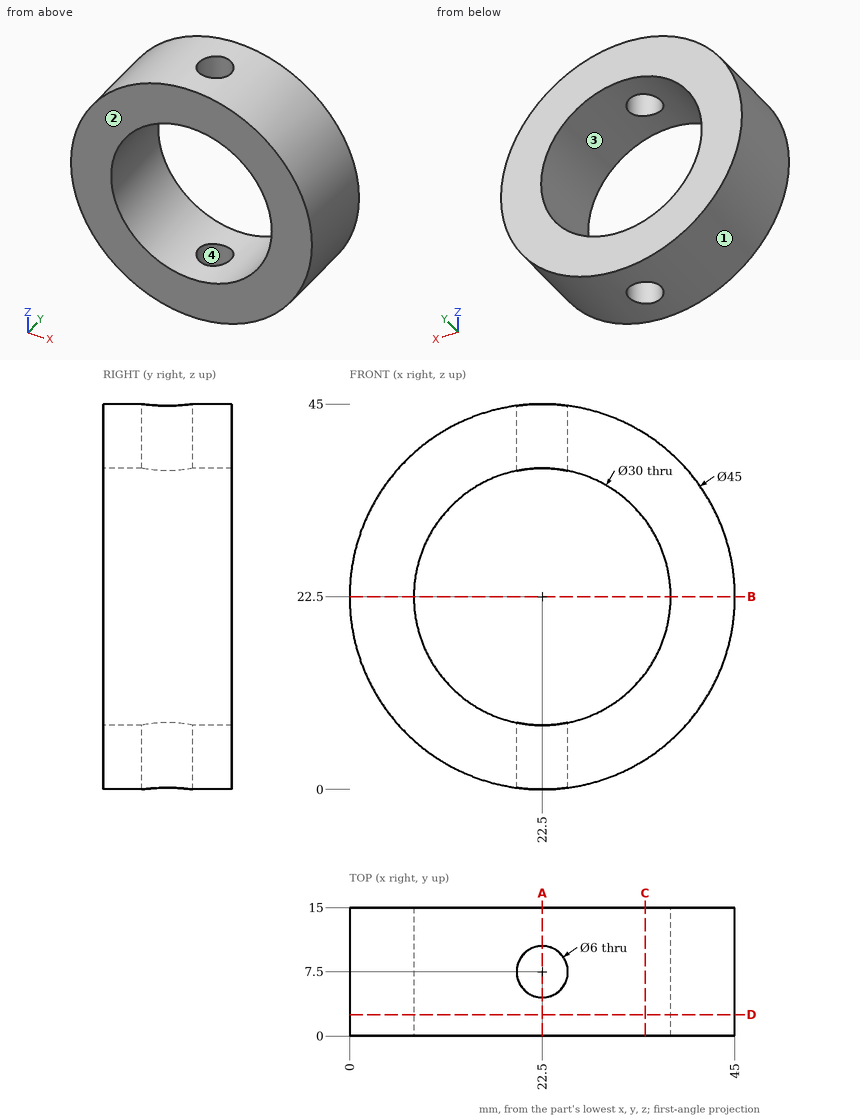
Study the drawing (mm; zero at the part's minimum x, y, z) and answer. Round coordinates to 2 decimals unless told otherwise and drop trailing zeros. Loops run counter-clockwise (first coordinate to the right, second up) from the corner with the lowest first, then second, coordinate; pieces in that order, holes last.
Q1. Find the intervals of material crossed by line 1 (Y direction, x = 22.5, z = 5); line 2 (X direction, y = 6.75, z = 17); line 3 (Y direction, x = 21.5, z = 37.5), in increasing order.
Q2. Given pin 1 Ø6 at (x, y) = (31.5, 8.5) entering from +Z; pin 2 Ø1 at (x, y) = (33, 7.5) entering from -Z; pin 3 Ø6 at (x, y) = (9.5, 8) entering from +Z, each flat-ended and moving along its own axis, determine where each tip first touches the part or whether it passes through.
Q3. Section C-C, the plane x = 34.5 is taken. Determine the outline of the cut face in (y, z).
Q4. Section A-A, the plane x = 22.5 is taken. Determine the outline of the cut face in (y, z), then the cut area to 3 significant figures.
Q5. Section B-B, the plane z = 22.5 is taken. Determine the outline of the cut face in (x, y).
Q6. For a pull along X with two mould halves and no side action, classify the marked faces 1, 2, 3 and 4 as released by +X, released by -X, zero draft, split by the parting line, or undercut.
Q7. Section D-D, the plane y = 2.5 is taken. Determine the outline of the cut face in (x, z), then the cut area to 3 significant figures.
Completed:
1. line 1: y = 0 to 4.5, 10.5 to 15
1. line 2: x = 0.68 to 8.54, 36.46 to 44.32
1. line 3: y = 0 to 4.67, 10.33 to 15
2. pin 1: stops at z = 44.19
2. pin 2: stops at z = 2.34
2. pin 3: stops at z = 42.66
3. outline: (0, 3.47) - (15, 3.47) - (15, 13.5) - (0, 13.5) - close; (0, 31.5) - (15, 31.5) - (15, 41.53) - (0, 41.53) - close
4. outline: (0, 0) - (4.5, 0) - (4.5, 7.5) - (0, 7.5) - close; (0, 37.5) - (4.5, 37.5) - (4.5, 45) - (0, 45) - close; (10.5, 0) - (15, 0) - (15, 7.5) - (10.5, 7.5) - close; (10.5, 37.5) - (15, 37.5) - (15, 45) - (10.5, 45) - close
4. area: 135 mm2
5. outline: (0, 0) - (7.5, 0) - (7.5, 15) - (0, 15) - close; (37.5, 0) - (45, 0) - (45, 15) - (37.5, 15) - close
6. face 1: split by the parting line
6. face 2: zero draft
6. face 3: undercut
6. face 4: undercut
7. outline: circle Ø45 at (22.5, 22.5); hole circle Ø30 at (22.5, 22.5)
7. area: 884 mm2
